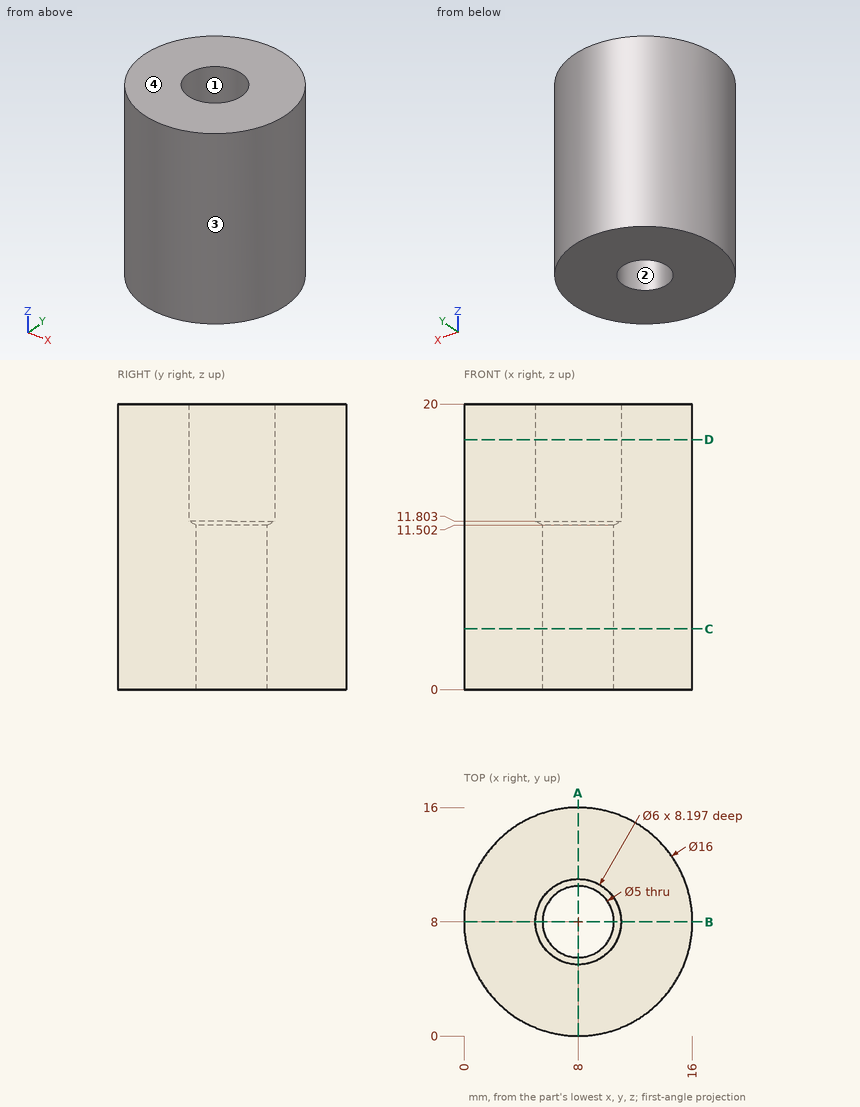
Can you work these out from the drawing? Everything is in mm from the part's minimum corner. Coordinates: 2 decimals unless noted, no trailing zeros. Write each loop counter-clockwise with the first axis right and the second up, starting at its lowest first coordinate (ties: lowest second). Pieces come first, ordered by that corner, then holes. Notation, with made-up numbers: (85, 14.5) -> (140, 14.5) arc R14 cw to (140, 31.5) -> close; hole circle Ø9 at (26, -15.5). An arc over 180 degrees is marked (long way). Write each question's results on one line, items separated by ' | '. Start each with the question number.
Item 1: If we section it at A-A, the plane x = 8: Write out the boundary of the cut face in (y, z), and give its area (3 significant figures).
Item 2: If we section it at D-D, the plane z = 17.5: Write out the boundary of the cut face in (x, y), and give its area (3 significant figures).
Item 3: Thinking about a two-plate mould opening in X: for the marked faces 1, 2, 3 and 4, which applies, released by +X, released by -X, zero draft, split by the parting line, or undercut?
Item 4: I'm going to push flat-ended pins straight in: P1, Ø4, axis at x = 8, y = 8, coming from the +Z side; P2, Ø6, axis at y = 3.5, z = 10.5, coming from the +X side. Where does each tip first touch, or does it pass through?
Item 5: Please list where these lines run through material, in increasing order: probe 1 along Y at (x, z) = (8, 18.25); probe 2 along X at (y, z) = (6, 1.5) (1 decimal); probe 3 along X at (y, z) = (9, 15.5).
Item 6: If we section it at C-C, the plane z = 4.25: Write out the boundary of the cut face in (x, y), and give its area (3 significant figures).
Answer block:
1) outline: (0, 0) -> (5.5, 0) -> (5.5, 11.5) -> (5, 11.8) -> (5, 20) -> (0, 20) -> close; (10.5, 0) -> (16, 0) -> (16, 20) -> (11, 20) -> (11, 11.8) -> (10.5, 11.5) -> close | area: 212 mm²
2) outline: circle Ø16 at (8, 8); hole circle Ø6 at (8, 8) | area: 173 mm²
3) face 1: undercut | face 2: undercut | face 3: split by the parting line | face 4: zero draft
4) P1: through | P2: x = 15.86
5) probe 1: 0 to 5, 11 to 16 | probe 2: 0.3 to 6.5, 9.5 to 15.7 | probe 3: 0.06 to 5.17, 10.83 to 15.94
6) outline: circle Ø16 at (8, 8); hole circle Ø5 at (8, 8) | area: 181 mm²
